Read the model definition and answer for the solid it produces. Units are mm, in the model's axes. A direction names the side the tool comes from. Give positions to 0.01 mm unless a question says otherwise; leave off trailing zeros. Write each loop counter-clockwise with the first axis right and the second up, starting at its lowest first coordinate (ties: lowest second). Pieces come first, ordered by that corner, then holes. Notation, with made-up numbers: M 57.25,55 L 63.25,55 A26 cw 63.25,91 Z; hole C -38.75,-18.75 d4. An arc over 180 degrees is marked long. Use a Markdown table: item, result. Add a question column.
Item 1: The mould has two halves that part along Y. Classify faces 4 (the cylindrical face through (2.535, -4.956, 15.738)), 5 (the flat face through (0, 7, -7)), 6 (the flat face through (3, -10.8, 0)): pulls with the +Y half, pulls with the -Y half, needs draft (parallel to the pull), parting line crosses it, or undercut.
Item 2: A cutting plane is placed at C-C on x = 2. Determine the outline of the cut face in (y, z), then the cut area to 3 significant figures.
Item 3: For faces 1 (the cylindrical face through (6.01, 13.18, -2.93)), 2 (the flat face through (3.5, -8.9, 2.2)), 3 (the flat face through (7, 9, 3)), determine the directions among +Z, -Z, +X, -X, +Y, -Y from which every point of the face is accessible in a straight line to the end or side of a thin tool.
Item 4: A cutting plane is placed at D-D on z = 11.5. Determine the outline of the cut face in (x, y).
Item 5: A cutting plane is placed at B-B on y = 0. Determine the outline of the cut face in (x, z).
Item 6: Consider probe 1 along Y at (x, z) = (4, 0); probe 2 along Z at (x, y) = (1.5, -8); probe 3 along Y at (x, z) = (4.5, -4). Determine where each line is inside the solid, lowest interval first. Write a range as [from, to].
Item 7: Given P1, Ø1.5, axis at x = 4.5, y = -10, coming from the +Z side; P2, Ø0.5, axis at x = 4.5, z = 2, coming from the -Y side; P3, Ø0.6, axis at x = 5, y = -10, coming from the -Z side, each flat-ended and moving along its own axis, determine where each tip first touches the part or whether it passes through.
Item 8: A cutting plane is placed at A-A on z = 0. Determine the outline of the cut face in (x, y).
from build123d import *

# Parameters (mm, degrees)
SKETCH_2_W        = 6
SKETCH_2_H        = 1.9
F_02_KEYWAY_DEPTH = 25.36185543


with BuildPart() as part:
    # 草图1 → 旋转1 (revolve)
    with BuildSketch(Plane.XY, mode=Mode.PRIVATE) as revolve_1_sk:
        Polygon((0, 9), (0, 16.5), (5, 16.5), (5, 13.5), (7, 13.5), (7, 9), align=None)
    revolve(revolve_1_sk.sketch.rotate(Axis((-3, 0, 0), (1, 0, 0)), 90), axis=Axis((-3, 0, 0), (1, 0, 0)))

    # 草图2 → 02_KEYWAY (cut, through all)
    with BuildSketch(Plane(origin=(0, 0, 0), x_dir=(0, 0, -1), z_dir=(1, 0, 0))):
        with Locations((0, -9.85)):
            Rectangle(SKETCH_2_W, SKETCH_2_H)
    extrude(amount=F_02_KEYWAY_DEPTH, mode=Mode.SUBTRACT)


solid = part.part
Filled in:
| question | item | result |
|---|---|---|
| 1 | face 4 | parting line crosses it |
| 1 | face 5 | needs draft |
| 1 | face 6 | undercut |
| 2 | outline | C 0,0 d33; hole M -10.8,-3 L -8.9,-3 L -8.9,-1.34 A9 ccw long -8.9,1.34 L -8.9,3 L -10.8,3 Z |
| 2 | area | 590 mm² |
| 3 | face 1 | +X |
| 3 | face 2 | +X, -X |
| 3 | face 3 | +Z, -Z, +X, +Y, -Y |
| 4 | outline | M 0,-11.83 L 5,-11.83 L 5,-7.07 L 7,-7.07 L 7,7.07 L 5,7.07 L 5,11.83 L 0,11.83 Z |
| 5 | outline | M 0,-16.5 L 5,-16.5 L 5,-13.5 L 7,-13.5 L 7,-9 L 0,-9 Z; M 0,9 L 7,9 L 7,13.5 L 5,13.5 L 5,16.5 L 0,16.5 Z |
| 6 | probe 1 | [-16.5, -10.8], [9, 16.5] |
| 6 | probe 2 | [-14.43, -4.12], [4.12, 14.43] |
| 6 | probe 3 | [-16.01, -8.06], [8.06, 16.01] |
| 7 | P1 | z = 13.66 |
| 7 | P2 | y = -16.41 |
| 7 | P3 | z = -13.35 |
| 8 | outline | M 0,-16.5 L 5,-16.5 L 5,-13.5 L 7,-13.5 L 7,-10.8 L 0,-10.8 Z; M 0,9 L 7,9 L 7,13.5 L 5,13.5 L 5,16.5 L 0,16.5 Z |
